Source: CAD feature listing. Evaluate the final solid. Frame: model axes, mm. Round coordinates to 2 decimals unless told otherwise and drop trailing zeros. Loops run counter-clockwise (first coordinate to the right, second up) from the corner with the lowest first, then second, coordinate; pieces in that order, holes last.
(1) Section B-B, the plane y = 993. Return the cut outline in (x, z), plus the area to 3 significant figures.
(2) Section A-A, the plane x = 529. Return the cut outline in (y, z).
(3) Material intervals for probe 1 along X at (y, z) = (768.35, 4.5); probe 2 along Y at (x, z) = (466.5, 5.5); probe 3 along X at (y, z) = (960.5, 4.5), sorted ascending.
(4) Section C-C, the plane z = 5. Count the separate pieces of the cut face and the enclosed holes in it, plus the area to 3 significant figures.
(5) First-contact query: pin 1 Ø4 at (x, y) = (269.875, 1047.75) entering from +Z; pin 2 Ø3 at (y, z) = (981.5, 3) entering from -X. Flat tips, straight axial feed; report the tip coordinate or a pass-through.
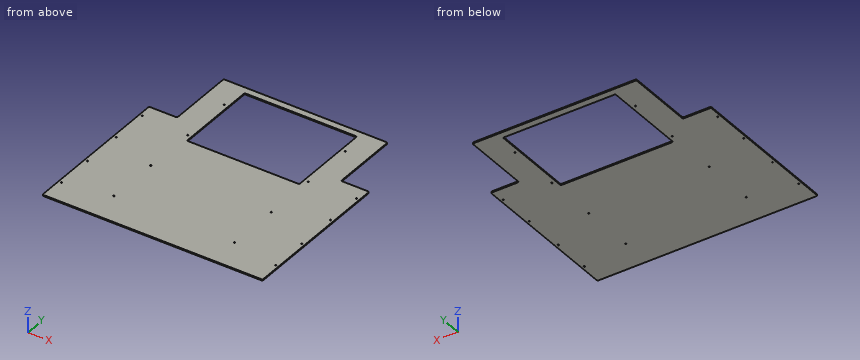
```python
from build123d import *

# Parameters (mm, degrees)
SKETCH1_W                   = 1193.8
SKETCH1_H                   = 1212.85
BOSS_EXTRUDE1_DEPTH         = 6.35
SKETCH2_W                   = 609.6
SKETCH2_H                   = 457.2
CUT_EXTRUDE1_DEPTH          = 1702.823693865
SKETCH3_W                   = 152.4
SKETCH3_H                   = 330.2
CUT_EXTRUDE2_DEPTH          = 1702.823693865
F_1_4_0_25_DIAMETER_HOLE1_D = 6.35
F_1_4_CLEARANCE_HOLE1_D     = 6.7564
SKETCH8_W                   = 152.4
SKETCH8_H                   = 38.1
CUT_EXTRUDE3_DEPTH          = 1702.823693865
FILLET1_R                   = 6.35


with BuildPart() as part:
    # Sketch1 → Boss-Extrude1 (new body)
    with BuildSketch(Plane.XY):
        with Locations((596.9, 606.425)):
            Rectangle(SKETCH1_W, SKETCH1_H)
    extrude(amount=BOSS_EXTRUDE1_DEPTH)

    # Sketch2 → Cut-Extrude1 (cut, through all)
    with BuildSketch(Plane.XY.offset(6.35)):
        with Locations((596.9, 946.15)):
            Rectangle(SKETCH2_W, SKETCH2_H)
    extrude(amount=-CUT_EXTRUDE1_DEPTH, mode=Mode.SUBTRACT)

    # Sketch3 → Cut-Extrude2 (cut, through all)
    with BuildSketch(Plane.XY.offset(6.35)):
        with Locations((76.2, 1009.65)):
            Rectangle(SKETCH3_W, SKETCH3_H)
        with Locations((1117.6, 1009.65)):
            Rectangle(SKETCH3_W, SKETCH3_H)
    extrude(amount=-CUT_EXTRUDE2_DEPTH, mode=Mode.SUBTRACT)

    # 1/4 (0.25) Diameter Hole1 (through all)
    with Locations(Plane.XY.offset(6.35)):
        with Locations((15.875, 127), (15.875, 333.375), (15.875, 561.975), (15.875, 768.35), (1177.925, 768.35), (1177.925, 561.975), (1177.925, 333.375), (1177.925, 127)):
            Hole(F_1_4_0_25_DIAMETER_HOLE1_D / 2)

    # 1/4 Clearance Hole1 (through all)
    with Locations(Plane.XY.offset(6.35)):
        with Locations((923.925, 1047.75), (269.875, 1047.75), (269.875, 755.65), (269.875, 463.55), (269.875, 171.45), (923.925, 171.45), (923.925, 463.55), (923.925, 755.65)):
            Hole(F_1_4_CLEARANCE_HOLE1_D / 2)

    # Sketch8 → Cut-Extrude3 (cut, through all)
    with BuildSketch(Plane.XY.offset(6.35)):
        with Locations((76.2, 1193.8)):
            Rectangle(SKETCH8_W, SKETCH8_H)
        with Locations((1117.6, 1193.8)):
            Rectangle(SKETCH8_W, SKETCH8_H)
    extrude(amount=-CUT_EXTRUDE3_DEPTH, mode=Mode.SUBTRACT)

    # Fillet1
    fillet1_edges = [part.edges().sort_by_distance(p)[0] for p in [
        (152.4, 1212.85, 3.175),
        (1041.4, 1212.85, 3.175),
        (292.1, 717.55, 3.175),
        (292.1, 1174.75, 3.175),
        (901.7, 1174.75, 3.175),
        (901.7, 717.55, 3.175),
        (0, 844.55, 3.175),
        (152.4, 844.55, 3.175),
        (1193.8, 844.55, 3.175),
        (1041.4, 844.55, 3.175),
        (1193.8, 0, 3.175),
        (0, 0, 3.175),
    ]]
    fillet(fillet1_edges, radius=FILLET1_R)


solid = part.part
```
Output values:
1. outline: (152.4, 0) - (292.1, 0) - (292.1, 6.35) - (152.4, 6.35) - close; (901.7, 0) - (1041.4, 0) - (1041.4, 6.35) - (901.7, 6.35) - close
1. area: 1,770 mm2
2. outline: (0, 0) - (717.55, 0) - (717.55, 6.35) - (0, 6.35) - close; (1174.75, 0) - (1212.85, 0) - (1212.85, 6.35) - (1174.75, 6.35) - close
3. probe 1: x = 0 to 12.7, 19.05 to 292.1, 901.7 to 1174.75, 1181.1 to 1193.8
3. probe 2: y = 0 to 717.55, 1174.75 to 1212.85
3. probe 3: x = 152.4 to 292.1, 901.7 to 1041.4
4. separate pieces: 1
4. enclosed holes: 17
4. area: 1,060,000 mm2
5. pin 1: passes through
5. pin 2: stops at x = 152.4
